Read the model definition and answer for the solid it produces. Units are mm, in the model's axes. A direction names the side the tool comes from. Coordinates: 2 decimals unless noted, no trailing zeros. Order: outer loops, then holes, each group sorted by start corner. A loop starts at its lowest first (then second) coordinate and runs counter-clockwise, first axis right, second up.
from build123d import *

# Parameters (mm, degrees)
SKETCH1_R           = 15.875
BOSS_EXTRUDE1_DEPTH = 215.9
SKETCH4_R           = 15.875
SKETCH4_R_2         = 12.588875
CUT_EXTRUDE3_DEPTH  = 69.85
CUT_EXTRUDE4_START  = -38.1
SKETCH5_R           = 15.875
SKETCH5_R_2         = 12.588875
CUT_EXTRUDE4_DEPTH  = 38.1
SKETCH7_R           = 12.588875
BOSS_EXTRUDE2_DEPTH = 38.1
SKETCH8_W           = 6.35
SKETCH8_H           = 6.477
CUT_EXTRUDE5_DEPTH  = 25.4
SKETCH9_R           = 12.588875
CUT_EXTRUDE6_DEPTH  = 25.4


with BuildPart() as part:
    # Sketch1 → Boss-Extrude1 (new, symmetric)
    with BuildSketch(Plane(origin=(0, 0, 0), x_dir=(1, 0, 0), z_dir=(0, 1, 0))):
        with Locations(Location((0, 0, 0), (0, 0, 270))):
            Circle(SKETCH1_R)
    extrude(amount=BOSS_EXTRUDE1_DEPTH, both=True)

    # Sketch4 → Cut-Extrude3 (cut)
    with BuildSketch(Plane(origin=(0, 215.9, 0), x_dir=(1, 0, 0), z_dir=(0, 1, 0))):
        with Locations(Location((0, 0, 0), (0, 0, 270))):
            Circle(SKETCH4_R)
        with Locations(Location((0, 0, 0), (0, 0, 270))):
            Circle(SKETCH4_R_2, mode=Mode.SUBTRACT)
    extrude(amount=-CUT_EXTRUDE3_DEPTH, mode=Mode.SUBTRACT)

    # Sketch5 → Cut-Extrude4 (cut)
    with BuildSketch(Plane.XZ.offset(215.9).offset(CUT_EXTRUDE4_START)):
        with Locations(Location((0, 0, 0), (0, 0, 270))):
            Circle(SKETCH5_R)
        with Locations(Location((0, 0, 0), (0, 0, 90))):
            Circle(SKETCH5_R_2, mode=Mode.SUBTRACT)
    extrude(amount=CUT_EXTRUDE4_DEPTH, mode=Mode.SUBTRACT)

    # Sketch7 → Boss-Extrude2 (add)
    with BuildSketch(Plane.XZ.offset(215.9)):
        with Locations(Location((0, 0, 0), (0, 0, 90))):
            Circle(SKETCH7_R)
    extrude(amount=BOSS_EXTRUDE2_DEPTH)

    # Sketch8 → Cut-Extrude5 (cut)
    with BuildSketch(Plane.XZ.offset(254)):
        with Locations((0, 12.468225)):
            Rectangle(SKETCH8_W, SKETCH8_H)
    extrude(amount=-CUT_EXTRUDE5_DEPTH, mode=Mode.SUBTRACT)

    # Sketch9 → Cut-Extrude6 (cut)
    with BuildSketch(Plane(origin=(0, 215.9, 0), x_dir=(1, 0, 0), z_dir=(0, 1, 0))):
        with Locations(Location((0, 0, 0), (0, 0, 270))):
            Circle(SKETCH9_R)
    extrude(amount=-CUT_EXTRUDE6_DEPTH, mode=Mode.SUBTRACT)


solid = part.part
Q1. Which of the six approach directions +Z, -Z, +X, -X, +Y, -Y give full straight-line access (tool end or side, diameter ignored) to faces 1 (the cylindrical face through (-12.48, -215.37, -1.64)), 2 (the flat face through (12, 146.05, -5)), 3 (the flat face through (0, 190.5, 0))?
Q2. Straight lines are drawn through the part: L1, parallel to Z at x = -1, y = -73; L2, parallel to Y at x = -3.5, z = 12.5. For each, find the intervals that lie inside material, in ascending order.
Q3. The part is cut by section C-C, the plane y = -12.5. Determine the outline of the cut face in (x, z) (3 decimals), then the cut area to 3 significant figures.
Q4. Each of these flat-tipped pins is pushed along its axis until it touches: P1, Ø1.5, axis at x = 5.5, y = 63, coming from the -Z side; P2, Ø3, axis at y = -18, z = 3, coming from the -X side; P3, Ø3, axis at y = 59.5, z = 4.5, coming from the +X side. Where does it stop, or does it pass through?
Q5. The part is cut by section B-B, the plane x = -9. Determine the outline of the cut face in (y, z).
Q6. The part is cut by section A-A, the plane z = 0. Determine the outline of the cut face in (x, y) (3 decimals).
Computed values:
1. face 1: -Y
1. face 2: +Y
1. face 3: +Z, -Z, +X, -X, +Y
2. L1: z = -15.84 to 15.84
2. L2: y = -177.8 to 146.05
3. outline: circle Ø31.75 at (0, 0)
3. area: 792 mm2
4. P1: stops at z = -15.15
4. P2: stops at x = -15.8
4. P3: stops at x = 15.59
5. outline: (-254, -8.8) - (-177.8, -8.8) - (-177.8, -13.08) - (146.05, -13.08) - (146.05, -8.8) - (190.5, -8.8) - (190.5, 8.8) - (146.05, 8.8) - (146.05, 13.08) - (-177.8, 13.08) - (-177.8, 8.8) - (-254, 8.8) - close
6. outline: (-15.875, -177.8) - (-12.589, -177.8) - (-12.589, -254) - (12.589, -254) - (12.589, -177.8) - (15.875, -177.8) - (15.875, 146.05) - (12.589, 146.05) - (12.589, 190.5) - (-12.589, 190.5) - (-12.589, 146.05) - (-15.875, 146.05) - close
